Could you check a few things on this model? Use its own coordinates, in mm. A direction names the side the tool comes from. Round coordinates to 2 decimals unless told otherwise and drop trailing zeros. Write each loop counter-clockwise with the first axis right and the second up, starting at its lowest first coordinate (ties: lowest second). Pieces come first, ordered by that corner, then holes. Notation, with made-up numbers: (23.5, 49) -> (79.5, 49) arc R22 ccw to (79.5, 86) -> close; hole circle Ø3 at (83, -6). An arc over 180 degrees is marked (long way). Answer in a Markdown table with one row per item.
from build123d import *

# Parameters (mm, degrees)
SKETCH1_W               = 20
SKETCH1_H               = 3
CUT_EXTRUDE1_DEPTH      = 14.472308498
CUT_EXTRUDE1_DEPTH_BACK = 14.472308498
SKETCH2_W               = 5.5
SKETCH2_H               = 3
SKETCH4_R               = 1.25
CUT_EXTRUDE2_DEPTH      = 3.2


with BuildPart() as part:
    # Sketch1 → Revolve1 (revolve)
    with BuildSketch(Plane.XY, mode=Mode.PRIVATE) as revolve1_sk:
        with Locations((1.095890411, 2.52739726)):
            Rectangle(SKETCH1_W, SKETCH1_H)
    revolve(revolve1_sk.sketch.rotate(Axis((-8.904109589, 4.02739726, 0), (1, 0, 0)), 270), axis=Axis((-8.904109589, 4.02739726, 0), (1, 0, 0)))

    # Sketch2 → Cut-Extrude1 (cut, two sides: drawn at the far end of the back side and taken through both)
    with BuildSketch(Plane.XY.offset(-CUT_EXTRUDE1_DEPTH_BACK)):
        with Locations((-6.154109589, 5.52739726)):
            Rectangle(SKETCH2_W, SKETCH2_H)
    extrude(amount=CUT_EXTRUDE1_DEPTH + CUT_EXTRUDE1_DEPTH_BACK, mode=Mode.SUBTRACT)

    # Sketch4 → Cut-Extrude2 (cut)
    with BuildSketch(Plane.XY.offset(3)):
        with Locations((0.095890411, 4.02739726)):
            Circle(SKETCH4_R)
    extrude(amount=-CUT_EXTRUDE2_DEPTH, mode=Mode.SUBTRACT)


solid = part.part
1) For faces 4 (the face through (-8.904, 3, 0)), 5 (the face through (0, 4, -0.2)), which set-ups out of +Z, -Z, +X, -X, +Y, -Y let a thin tool reach every point of the face, with its end or its side?
Findings:
| item | result |
|---|---|
| face 4 | +Z, -Z, -X, +Y, -Y |
| face 5 | +Z |
2) Please list where these lines run through material, in increasing order: line 1 (X direction, y = 6, z = -1.75); line 2 (X direction, y = 4.25, z = 0); line 3 (Y direction, x = 7, z = 2.25).
Findings:
| item | result |
|---|---|
| line 1 | x = -3.4 to 11.1 |
| line 2 | x = -3.4 to -1.13, 1.33 to 11.1 |
| line 3 | y = 2.04 to 6.01 |
3) Thinking about a two-plate mould opening in Y: for faces 1 (the face through (-6, 4.027, 0)), 2 (the face through (-1.153, 4.082, 1.422)), 3 (the face through (-3.404, 5, 0)), which applies, +Y half, -Y half, draft (parallel to the pull), parting line (faces both ways), or undercut?
Findings:
| item | result |
|---|---|
| face 1 | +Y half |
| face 2 | undercut |
| face 3 | draft |
4) Imagine slicing it at C-C, the plane x = -7. Please give me the cut outline in (y, z).
Findings:
| item | result |
|---|---|
| outline | (4.03, -3) -> (4.03, 3) arc R3 ccw to start |
5) Imagine slicing it at D-D, the plane z = 1.75. Please give me the cut outline in (x, y), plus the area to 3 significant figures.
Findings:
| item | result |
|---|---|
| outline | (-8.9, 1.59) -> (11.1, 1.59) -> (11.1, 6.46) -> (-3.4, 6.46) -> (-3.4, 4.03) -> (-8.9, 4.03) -> close; hole circle Ø2.5 at (0.1, 4.03) |
| area | 79.2 mm^2 |
6) Imagine slicing it at B-B, the plane y = 3.5. Please give me the cut outline in (x, z).
Findings:
| item | result |
|---|---|
| outline | (-8.9, -2.95) -> (11.1, -2.95) -> (11.1, 2.95) -> (1.23, 2.95) -> (1.23, -0.2) -> (-1.04, -0.2) -> (-1.04, 2.95) -> (-8.9, 2.95) -> close |
7) For pin 1 (0.8 mm diameter, centred on x = -0.5, y = 4.5, fed in from +Z); pin 2 (2.5 mm diameter, centred on y = 6, z = 0.5, fed in from -X), each with a flat end and sliding along its axis, tell me the tip position at first contact or that it passes through.
Findings:
| item | result |
|---|---|
| pin 1 | stops at z = -0.2 |
| pin 2 | stops at x = -3.4 |
8) Imagine slicing it at A-A, the plane z = 0. Please give me the cut outline in (x, y).
Findings:
| item | result |
|---|---|
| outline | (-8.9, 1.03) -> (11.1, 1.03) -> (11.1, 7.03) -> (-3.4, 7.03) -> (-3.4, 4.03) -> (-8.9, 4.03) -> close; hole circle Ø2.5 at (0.1, 4.03) |
